```python
from build123d import *

# Parameters (mm, degrees)
SALIENTE_EXTRUIR1_DEPTH = 60
CROQUIS5_W              = 68
CROQUIS5_H              = 44
CORTAR_EXTRUIR1_DEPTH   = 128.769323392
CHAFL_N1_SIZE           = 3
CROQUIS6_R              = 30
SALIENTE_EXTRUIR4_DEPTH = 6
CROQUIS7_R              = 15
SALIENTE_EXTRUIR5_DEPTH = 276
SALIENTE_EXTRUIR6_DEPTH = 30
CORTAR_EXTRUIR2_REACH   = 379.323
CROQUIS9_W              = 27.2
CROQUIS9_H              = 44
CORTAR_EXTRUIR3_DEPTH   = 60
SALIENTE_EXTRUIR7_REACH = 356.313
CROQUIS11_R             = 4
CROQUIS13_R             = 26
SALIENTE_EXTRUIR8_DEPTH = 5
CROQUIS14_R             = 10
SALIENTE_EXTRUIR9_DEPTH = 10.75
CROQUIS15_R             = 5
CORTAR_EXTRUIR4_DEPTH   = 371.451835601


with BuildPart() as part:
    # Croquis2 → Saliente-Extruir1 (new body)
    with BuildSketch(Plane(origin=(0, 0, 0), x_dir=(1, 0, 0), z_dir=(0, 1, 0))):
        with BuildLine():
            Line((-25, -23), (-25, 23))
            Line((-25, 23), (80, 23))
            ThreePointArc((80, 23), (103, 0), (80, -23))
            Line((80, -23), (-25, -23))
        make_face()
    extrude(amount=SALIENTE_EXTRUIR1_DEPTH)

    # Croquis5 → Cortar-Extruir1 (cut, through all)
    with BuildSketch(Plane.XY.offset(23)):
        with Locations((69, 30)):
            Rectangle(CROQUIS5_W, CROQUIS5_H)
    extrude(amount=-CORTAR_EXTRUIR1_DEPTH, mode=Mode.SUBTRACT)

    # Chaflán1
    chafl_n1_edges = [part.edges().sort_by_distance(p)[0] for p in [
        (-25, 60, 0),
        (-25, 0, 0),
    ]]
    chamfer(chafl_n1_edges, length=CHAFL_N1_SIZE)

    # Croquis6 → Saliente-Extruir4 (add)
    with BuildSketch(Plane.XY.offset(23)):
        with Locations(Location((0, 30, 0), (0, 0, 146.442690238))):
            Circle(CROQUIS6_R)
    extrude(amount=SALIENTE_EXTRUIR4_DEPTH)

    # Croquis7 → Saliente-Extruir5 (add)
    with BuildSketch(Plane.XY.offset(29)):
        with Locations((0, 30)):
            Circle(CROQUIS7_R)
    extrude(amount=SALIENTE_EXTRUIR5_DEPTH)

    # Croquis8 → Saliente-Extruir6 (add)
    with BuildSketch(Plane.XY.offset(305)):
        Polygon((-22, 60), (55, 60), (55, 0), (-22, 0), (-25, 3), (-25, 57), align=None)
    extrude(amount=SALIENTE_EXTRUIR6_DEPTH)

    # Croquis9 → Cortar-Extruir2 (cut, up to next)
    with BuildSketch(Plane.XY.offset(335), mode=Mode.PRIVATE) as cortar_extruir2_sk1:
        with Locations((41.4, 30)):
            Rectangle(CROQUIS9_W, CROQUIS9_H)
    cortar_extruir2_tool1 = extrude(cortar_extruir2_sk1.sketch, amount=-CORTAR_EXTRUIR2_REACH, mode=Mode.PRIVATE) & part.part
    add(cortar_extruir2_tool1.solids().sort_by_distance((41.4, 30, 335))[0], mode=Mode.SUBTRACT)

    # Croquis10 → Cortar-Extruir3 (cut)
    with BuildSketch(Plane.XZ):
        with BuildLine():
            Line((55, 335), (27.8, 335))
            Line((27.8, 335), (47.605709584, 329.654546989))
            ThreePointArc((47.605709584, 329.654546989), (52.939052079, 326.080415453), (55, 320))
            Line((55, 320), (55, 335))
        make_face()
        with BuildLine():
            Line((55, 305), (55, 320))
            ThreePointArc((55, 320), (52.939052079, 313.919584547), (47.605709584, 310.345453011))
            Line((47.605709584, 310.345453011), (27.8, 305))
            Line((27.8, 305), (55, 305))
        make_face()
    extrude(amount=-CORTAR_EXTRUIR3_DEPTH, mode=Mode.SUBTRACT)

    # Croquis11 → Saliente-Extruir7 (add, up to next)
    with BuildSketch(Plane.XZ.offset(-52), mode=Mode.PRIVATE) as saliente_extruir7_sk1:
        with Locations(Location((45, 320, 0), (0, 0, 90))):
            Circle(CROQUIS11_R)
    saliente_extruir7_tool1 = extrude(saliente_extruir7_sk1.sketch, amount=SALIENTE_EXTRUIR7_REACH, mode=Mode.PRIVATE) - part.part
    add(saliente_extruir7_tool1.solids().sort_by_distance((45, 52, 320))[0])

    # Croquis13 → Saliente-Extruir8 (add)
    with BuildSketch(Plane.XY.offset(335)):
        with Locations(Location((1.4, 30, 0), (0, 0, 180))):
            Circle(CROQUIS13_R)
    extrude(amount=SALIENTE_EXTRUIR8_DEPTH)

    # Croquis14 → Saliente-Extruir9 (add)
    with BuildSketch(Plane.XY.offset(340)):
        with Locations((1.4, 30)):
            Circle(CROQUIS14_R)
    extrude(amount=SALIENTE_EXTRUIR9_DEPTH)

    # Croquis15 → Cortar-Extruir4 (cut, through all)
    with BuildSketch(Plane.XZ):
        with Locations(Location((80, 0, 0), (0, 0, 270))):
            Circle(CROQUIS15_R)
    extrude(amount=-CORTAR_EXTRUIR4_DEPTH, mode=Mode.SUBTRACT)


solid = part.part
```
For this review, take the finished solid that the model builds, in its own axes (mm). A direction names the side the tool comes from. Coordinates: 2 decimals unless noted, no trailing zeros. Write each loop counter-clockwise with the first axis right and the second up, starting at its lowest first coordinate (ties: lowest second). Pieces come first, ordered by that corner, then holes. Notation, with made-up numbers: (81.5, 26) -> (92.5, 26) arc R6 ccw to (92.5, 33) -> close; hole circle Ø4 at (-8, 58.25). An arc over 180 degrees is marked (long way). Put each result on its own line as item: value.
Q1. Tool access review of faces 4 (the flat face through (-25, 30, 0)), 5 (the flat face through (35, 30, 0)), 6 (the flat face through (-19, 4, 23)), 7 (the cylindrical face through (21.61, 50.81, 25.96)): name each direction out of +Z, -Z, +X, -X, +Y, -Y from which nothing blocks a thin tool from reaching the whole face with its end or side.
From the geometry:
face 4: -Z, -X, +Y, -Y
face 5: +Z, -Z, +X
face 6: -X, -Y
face 7: none
Q2. Wall thickness on L1, parallel to X at y = 3.75, z = 0; L2, parallel to Z at x = -8.5, y = 50.5; L3, parallel to X at y = 19.5, z = 333: over which ranges is each line inside the solid? List them lowest first.
From the geometry:
L1: x = -25 to 75, 85 to 103
L2: z = -23 to 29, 305 to 340
L3: x = -25 to 27.8
Q3. Take a section at B-B, the plane x = 4. State the section outline as (y, z) points, then the cut area to 3 significant figures.
From the geometry:
outline: (0, -23) -> (60, -23) -> (60, 23) -> (59.73, 23) -> (59.73, 29) -> (44.46, 29) -> (44.46, 305) -> (60, 305) -> (60, 335) -> (55.87, 335) -> (55.87, 340) -> (39.66, 340) -> (39.66, 350.75) -> (20.34, 350.75) -> (20.34, 340) -> (4.13, 340) -> (4.13, 335) -> (0, 335) -> (0, 305) -> (15.54, 305) -> (15.54, 29) -> (0.27, 29) -> (0.27, 23) -> (0, 23) -> close
area: 13,400 mm2
Q4. The part is to be moulded in two halves that separate along Z. For faces 1 (the flat face through (17, 0, 320)), 2 (the cylindrical face through (75.12, 3.94, 1.08)), 3 (the cylindrical face through (102.994, 3.944, -0.506)), say which applies: +Z half, -Z half, draft (parallel to the pull), parting line (faces both ways), or undercut.
From the geometry:
face 1: draft
face 2: undercut
face 3: parting line
Q5. Clearance check with flat-ended pins moving along their axes: pin 1 Ø4 at (y, z) = (45.5, 142.5) entering from -X; pin 2 Ø15 at (y, z) = (17, 325.5) entering from -X; pin 3 Ø3 at (y, z) = (40, 102.5) entering from +X. State where each tip first meets the part, or that it passes through.
From the geometry:
pin 1: stops at x = -6.54
pin 2: stops at x = -25
pin 3: stops at x = 12.36
Q6. Take a section at C-C, the plane z = 162.5. State the section outline as (x, y) points.
From the geometry:
outline: circle Ø30 at (0, 30)
Q7. Take a section at A-A, the plane y = 30. State the section outline as (x, z) points.
From the geometry:
outline: (-30, 23) -> (-25, 23) -> (-25, -23) -> (35, -23) -> (35, 23) -> (30, 23) -> (30, 29) -> (15, 29) -> (15, 305) -> (27.8, 305) -> (27.8, 335) -> (27.4, 335) -> (27.4, 340) -> (11.4, 340) -> (11.4, 350.75) -> (-8.6, 350.75) -> (-8.6, 340) -> (-24.6, 340) -> (-24.6, 335) -> (-25, 335) -> (-25, 305) -> (-15, 305) -> (-15, 29) -> (-30, 29) -> close; circle Ø8 at (45, 320)
